The listing builds one solid part. Answer for the finished solid, in the listing's coordinates (mm). A direction names the side the tool comes from. Coordinates: 2 decimals unless noted, no trailing zeros. Order: outer loops, then holes, each group sorted by start corner. A loop starts at its lowest first (then second) coordinate and runs counter-clockwise, first axis right, second up. Notation, with made-up numbers: (-15, 35.5) -> (34, 35.5) arc R23 cw to (34, 70.5) -> close; hole circle Ø5 at (-1, 78.25). An arc over 180 degrees is marked (long way). Return JSON: item names as keys, results as strings.
from build123d import *

# Parameters (mm, degrees)
CUT_EXTRUDE1_REACH = 211.949
SKETCH2_R          = 2
CUT_EXTRUDE2_REACH = 211.949
SKETCH3_R          = 2


with BuildPart() as part:
    # Sketch1 → Revolve4 (revolve)
    with BuildSketch(Plane.XY, mode=Mode.PRIVATE) as revolve4_sk:
        with BuildLine():
            Line((80, 1.161847476), (76.618474759, 10.572760664))
            Line((76.618474759, 10.572760664), (80, 19.983673853))
            Line((80, 19.983673853), (76.618474759, 29.394587041))
            Line((76.618474759, 29.394587041), (80, 38.80550023))
            Line((80, 38.80550023), (76.618474759, 48.216413418))
            Line((76.618474759, 48.216413418), (80, 57.627326607))
            Line((80, 57.627326607), (76.618474759, 67.038239796))
            Line((76.618474759, 67.038239796), (80, 76.449152984))
            Line((80, 76.449152984), (76.618474759, 85.860066173))
            Line((76.618474759, 85.860066173), (80, 95.270979361))
            Line((80, 95.270979361), (76.618474759, 104.68189255))
            Line((76.618474759, 104.68189255), (80, 114.092805738))
            Line((80, 114.092805738), (76.618474759, 123.503718927))
            Line((76.618474759, 123.503718927), (80, 132.914632115))
            Line((80, 132.914632115), (76.618474759, 142.325545304))
            Line((76.618474759, 142.325545304), (80, 151.736458492))
            Line((80, 151.736458492), (34.99586215, 151.736458492))
            Line((34.99586215, 151.736458492), (34.99586215, 154.736458492))
            ThreePointArc((34.99586215, 154.736458492), (35.99586215, 155.736458492), (34.99586215, 156.736458492))
            Line((34.99586215, 156.736458492), (97.843831402, 156.736458492))
            Line((97.843831402, 156.736458492), (97.843831402, 153.736458492))
            Line((97.843831402, 153.736458492), (82.843831406, 153.736458492))
            Line((82.843831406, 153.736458492), (78.743667033, 142.325545304))
            Line((78.743667033, 142.325545304), (82.125192274, 132.914632115))
            Line((82.125192274, 132.914632115), (78.743667033, 123.503718927))
            Line((78.743667033, 123.503718927), (82.125192274, 114.092805738))
            Line((82.125192274, 114.092805738), (78.743667033, 104.68189255))
            Line((78.743667033, 104.68189255), (82.125192274, 95.270979361))
            Line((82.125192274, 95.270979361), (78.743667033, 85.860066173))
            Line((78.743667033, 85.860066173), (82.125192274, 76.449152984))
            Line((82.125192274, 76.449152984), (78.743667033, 67.038239796))
            Line((78.743667033, 67.038239796), (82.125192274, 57.627326607))
            Line((82.125192274, 57.627326607), (78.743667033, 48.216413418))
            Line((78.743667033, 48.216413418), (82.125192274, 38.80550023))
            Line((82.125192274, 38.80550023), (78.743667033, 29.394587041))
            Line((78.743667033, 29.394587041), (82.125192274, 19.983673853))
            Line((82.125192274, 19.983673853), (78.743667033, 10.572760664))
            Line((78.743667033, 10.572760664), (81.882182638, 1.838152524))
            Line((81.882182638, 1.838152524), (95, 1.838152524))
            Line((95, 1.838152524), (95, -1.161847476))
            Line((95, -1.161847476), (65, -1.161847476))
            Line((65, -1.161847476), (65, 1.161847476))
            Line((65, 1.161847476), (80, 1.161847476))
        make_face()
    revolve(revolve4_sk.sketch.rotate(Axis((0, 0, 0), (0, 1, 0)), 90), axis=Axis((0, 0, 0), (0, 1, 0)))

    # Sketch2 → Cut-Extrude1 (cut, up to next)
    with BuildSketch(Plane(origin=(0, 156.736458492, 0), x_dir=(1, 0, 0), z_dir=(0, 1, 0)), mode=Mode.PRIVATE) as cut_extrude1_sk1:
        with Locations(Location((-85.928885632, 13.609798458, 0), (0, 0, 270))):
            Circle(SKETCH2_R)
    cut_extrude1_tool1 = extrude(cut_extrude1_sk1.sketch, amount=-CUT_EXTRUDE1_REACH, mode=Mode.PRIVATE) & part.part
    # Sketch2 → Cut-Extrude1 (cut, up to next)
    with BuildSketch(Plane(origin=(0, 156.736458492, 0), x_dir=(1, 0, 0), z_dir=(0, 1, 0)), mode=Mode.PRIVATE) as cut_extrude1_sk2:
        with Locations(Location((-85.928885632, -13.609798458, 0), (0, 0, 270))):
            Circle(SKETCH2_R)
    cut_extrude1_tool2 = extrude(cut_extrude1_sk2.sketch, amount=-CUT_EXTRUDE1_REACH, mode=Mode.PRIVATE) & part.part
    # Sketch2 → Cut-Extrude1 (cut, up to next)
    with BuildSketch(Plane(origin=(0, 156.736458492, 0), x_dir=(1, 0, 0), z_dir=(0, 1, 0)), mode=Mode.PRIVATE) as cut_extrude1_sk3:
        with Locations(Location((85.928885632, 13.609798458, 0), (0, 0, 270))):
            Circle(SKETCH2_R)
    cut_extrude1_tool3 = extrude(cut_extrude1_sk3.sketch, amount=-CUT_EXTRUDE1_REACH, mode=Mode.PRIVATE) & part.part
    # Sketch2 → Cut-Extrude1 (cut, up to next)
    with BuildSketch(Plane(origin=(0, 156.736458492, 0), x_dir=(1, 0, 0), z_dir=(0, 1, 0)), mode=Mode.PRIVATE) as cut_extrude1_sk4:
        with Locations(Location((85.928885632, -13.609798458, 0), (0, 0, 270))):
            Circle(SKETCH2_R)
    cut_extrude1_tool4 = extrude(cut_extrude1_sk4.sketch, amount=-CUT_EXTRUDE1_REACH, mode=Mode.PRIVATE) & part.part
    # Sketch2 → Cut-Extrude1 (cut, up to next)
    with BuildSketch(Plane(origin=(0, 156.736458492, 0), x_dir=(1, 0, 0), z_dir=(0, 1, 0)), mode=Mode.PRIVATE) as cut_extrude1_sk5:
        with Locations(Location((-30, 81.663945533, 0), (0, 0, 270))):
            Circle(SKETCH2_R)
    cut_extrude1_tool5 = extrude(cut_extrude1_sk5.sketch, amount=-CUT_EXTRUDE1_REACH, mode=Mode.PRIVATE) & part.part
    # Sketch2 → Cut-Extrude1 (cut, up to next)
    with BuildSketch(Plane(origin=(0, 156.736458492, 0), x_dir=(1, 0, 0), z_dir=(0, 1, 0)), mode=Mode.PRIVATE) as cut_extrude1_sk6:
        with Locations(Location((30, 81.663945533, 0), (0, 0, 270))):
            Circle(SKETCH2_R)
    cut_extrude1_tool6 = extrude(cut_extrude1_sk6.sketch, amount=-CUT_EXTRUDE1_REACH, mode=Mode.PRIVATE) & part.part
    # Sketch2 → Cut-Extrude1 (cut, up to next)
    with BuildSketch(Plane(origin=(0, 156.736458492, 0), x_dir=(1, 0, 0), z_dir=(0, 1, 0)), mode=Mode.PRIVATE) as cut_extrude1_sk7:
        with Locations(Location((30, -81.663945533, 0), (0, 0, 270))):
            Circle(SKETCH2_R)
    cut_extrude1_tool7 = extrude(cut_extrude1_sk7.sketch, amount=-CUT_EXTRUDE1_REACH, mode=Mode.PRIVATE) & part.part
    # Sketch2 → Cut-Extrude1 (cut, up to next)
    with BuildSketch(Plane(origin=(0, 156.736458492, 0), x_dir=(1, 0, 0), z_dir=(0, 1, 0)), mode=Mode.PRIVATE) as cut_extrude1_sk8:
        with Locations(Location((-30, -81.663945533, 0), (0, 0, 270))):
            Circle(SKETCH2_R)
    cut_extrude1_tool8 = extrude(cut_extrude1_sk8.sketch, amount=-CUT_EXTRUDE1_REACH, mode=Mode.PRIVATE) & part.part
    add(cut_extrude1_tool1.solids().sort_by_distance((-85.928886, 156.736458, -13.609798))[0], mode=Mode.SUBTRACT)
    add(cut_extrude1_tool2.solids().sort_by_distance((-85.928886, 156.736458, 13.609798))[0], mode=Mode.SUBTRACT)
    add(cut_extrude1_tool3.solids().sort_by_distance((85.928886, 156.736458, -13.609798))[0], mode=Mode.SUBTRACT)
    add(cut_extrude1_tool4.solids().sort_by_distance((85.928886, 156.736458, 13.609798))[0], mode=Mode.SUBTRACT)
    add(cut_extrude1_tool5.solids().sort_by_distance((-30, 156.736458, -81.663946))[0], mode=Mode.SUBTRACT)
    add(cut_extrude1_tool6.solids().sort_by_distance((30, 156.736458, -81.663946))[0], mode=Mode.SUBTRACT)
    add(cut_extrude1_tool7.solids().sort_by_distance((30, 156.736458, 81.663946))[0], mode=Mode.SUBTRACT)
    add(cut_extrude1_tool8.solids().sort_by_distance((-30, 156.736458, 81.663946))[0], mode=Mode.SUBTRACT)

    # Sketch3 → Cut-Extrude2 (cut, up to next)
    with BuildSketch(Plane.XZ.offset(1.161847476), mode=Mode.PRIVATE) as cut_extrude2_sk1:
        with Locations(Location((0, 87, 0), (0, 0, 270))):
            Circle(SKETCH3_R)
    cut_extrude2_tool1 = extrude(cut_extrude2_sk1.sketch, amount=-CUT_EXTRUDE2_REACH, mode=Mode.PRIVATE) & part.part
    # Sketch3 → Cut-Extrude2 (cut, up to next)
    with BuildSketch(Plane.XZ.offset(1.161847476), mode=Mode.PRIVATE) as cut_extrude2_sk2:
        with Locations(Location((75.344210129, 43.5, 0), (0, 0, 270))):
            Circle(SKETCH3_R)
    cut_extrude2_tool2 = extrude(cut_extrude2_sk2.sketch, amount=-CUT_EXTRUDE2_REACH, mode=Mode.PRIVATE) & part.part
    # Sketch3 → Cut-Extrude2 (cut, up to next)
    with BuildSketch(Plane.XZ.offset(1.161847476), mode=Mode.PRIVATE) as cut_extrude2_sk3:
        with Locations(Location((75.344210129, -43.5, 0), (0, 0, 270))):
            Circle(SKETCH3_R)
    cut_extrude2_tool3 = extrude(cut_extrude2_sk3.sketch, amount=-CUT_EXTRUDE2_REACH, mode=Mode.PRIVATE) & part.part
    # Sketch3 → Cut-Extrude2 (cut, up to next)
    with BuildSketch(Plane.XZ.offset(1.161847476), mode=Mode.PRIVATE) as cut_extrude2_sk4:
        with Locations(Location((0, -87, 0), (0, 0, 270))):
            Circle(SKETCH3_R)
    cut_extrude2_tool4 = extrude(cut_extrude2_sk4.sketch, amount=-CUT_EXTRUDE2_REACH, mode=Mode.PRIVATE) & part.part
    # Sketch3 → Cut-Extrude2 (cut, up to next)
    with BuildSketch(Plane.XZ.offset(1.161847476), mode=Mode.PRIVATE) as cut_extrude2_sk5:
        with Locations(Location((-75.344210129, -43.5, 0), (0, 0, 270))):
            Circle(SKETCH3_R)
    cut_extrude2_tool5 = extrude(cut_extrude2_sk5.sketch, amount=-CUT_EXTRUDE2_REACH, mode=Mode.PRIVATE) & part.part
    # Sketch3 → Cut-Extrude2 (cut, up to next)
    with BuildSketch(Plane.XZ.offset(1.161847476), mode=Mode.PRIVATE) as cut_extrude2_sk6:
        with Locations(Location((-75.344210129, 43.5, 0), (0, 0, 270))):
            Circle(SKETCH3_R)
    cut_extrude2_tool6 = extrude(cut_extrude2_sk6.sketch, amount=-CUT_EXTRUDE2_REACH, mode=Mode.PRIVATE) & part.part
    add(cut_extrude2_tool1.solids().sort_by_distance((0, -1.161847, 87))[0], mode=Mode.SUBTRACT)
    add(cut_extrude2_tool2.solids().sort_by_distance((75.34421, -1.161847, 43.5))[0], mode=Mode.SUBTRACT)
    add(cut_extrude2_tool3.solids().sort_by_distance((75.34421, -1.161847, -43.5))[0], mode=Mode.SUBTRACT)
    add(cut_extrude2_tool4.solids().sort_by_distance((0, -1.161847, -87))[0], mode=Mode.SUBTRACT)
    add(cut_extrude2_tool5.solids().sort_by_distance((-75.34421, -1.161847, -43.5))[0], mode=Mode.SUBTRACT)
    add(cut_extrude2_tool6.solids().sort_by_distance((-75.34421, -1.161847, 43.5))[0], mode=Mode.SUBTRACT)


solid = part.part
1. Consider line 1 (Y direction, x = 3, z = 69); line 2 (X direction, y = 0, z = 43); line 3 (X direction, y = 14, z = -62). Determine where each line is inside the solid, lowest interval first. Write a range as from..to.
Answer block:
{"line 1": "y = -1.16..1.16, 151.74..156.74", "line 2": "x = -84.71..-77.28, -73.41..-48.74, 48.74..73.41, 77.28..84.71", "line 3": "x = -50.52..-47.08, 47.08..50.52"}
2. Determine the mould class of faces 3 (the face through (-80.2, 153.736, 22.2)), 4 (the face through (-23.063, 10.116, -73.237)), 5 (the face through (-23.72, 85.27, -75.31)) for opening direction Z: pulls with the +Z half, pulls with the -Z half, needs draft (parallel to the pull), parting line crosses it, or undercut.
Answer block:
{"face 3": "needs draft", "face 4": "undercut", "face 5": "parting line crosses it"}
3. Each of these flat-tipped pins is pushed along its axis until it touches: pin 1 Ø5 at (x, y) = (-55.5, 101) entering from -Z; pin 2 Ø12 at (y, z) = (89.5, 58) entering from -X; pin 3 Ø3.5 at (x, z) = (85.93, 13.61) entering from +Y. Where does it stop, or does it pass through?
Answer block:
{"pin 1": "stops at z = -60.32", "pin 2": "stops at x = -61.59", "pin 3": "stops at y = 1.84"}
4. The part is cut by section A-A on y = 43. Give the vertices of the cut face in (x, z).
Answer block:
{"outline": "circle Ø161.24 at (0, 0); hole circle Ø156.99 at (0, 0)"}
5. For faces 1 (the face through (-10.51, 153.26, -33.38)), 2 (the face through (75, 105.27, 16.66)), determine the directions among +Z, -Z, +X, -X, +Y, -Y from which every point of the face is accessible in a straight line to the end or side of a thin tool.
Answer block:
{"face 1": "+Y, -Y", "face 2": "none"}
6. The part is cut by section B-B on y = 119.5. Give the vertices of the cut face in (x, z).
Answer block:
{"outline": "circle Ø160.36 at (0, 0); hole circle Ø156.11 at (0, 0)"}
